from build123d import *

# Parameters (mm, degrees)
PROFILE_SKETCH_W               = 20
PROFILE_SKETCH_H               = 22
PROFILE_EXTRUDE_DEPTH          = 25
GUSSET_1_EXTRUDE_DEPTH         = 3
GUSSET_START                   = 22
GUSSET_2_EXTRUDE_DEPTH         = 3
SOLENOID_MOUNTING_HOLES_D      = 3.4
SOLENOID_MOUNTING_HOLES_DEPTH  = 3
NO_6_MOUNTING_HOLES_AT_2_COUNT = 2
NO_6_MOUNTING_HOLES_AT_2_PITCH = 10
FILLET3_R                      = 3
FILLET4_R                      = 2
FILLET5_R                      = 3
FILLET6_R                      = 1.5


with BuildPart() as part:
    # Profile Sketch → Profile  Extrude (new body)
    with BuildSketch(Plane.XY):
        Polygon((0, 0), (0, 25), (-26, 25), (-26, -4), (14, -4), (14, 0), align=None)
        with Locations((-13, 11)):
            Rectangle(PROFILE_SKETCH_W, PROFILE_SKETCH_H, mode=Mode.SUBTRACT)
    extrude(amount=PROFILE_EXTRUDE_DEPTH)

    # Gusset Sketch → Gusset 1 Extrude (add)
    with BuildSketch(Plane.XY):
        Polygon((0, 0), (14, 0), (0, 9), align=None)
    extrude(amount=GUSSET_1_EXTRUDE_DEPTH)

    # Gusset Sketch<2> → Gusset 2 Extrude (add)
    with BuildSketch(Plane.XY.offset(GUSSET_START)):
        Polygon((0, 0), (14, 0), (0, 9), align=None)
    extrude(amount=GUSSET_2_EXTRUDE_DEPTH)

    # Solenoid Mounting Holes
    with Locations(Plane(origin=(-25, 25, 0), x_dir=(0, 0, -1), z_dir=(0, 1, 0))):
        with Locations((-5, -17), (-20, -17), (-20, -7), (-5, -7)):
            Hole(SOLENOID_MOUNTING_HOLES_D / 2, depth=SOLENOID_MOUNTING_HOLES_DEPTH)

    # No. 6 Mounting Holes Profile Sketch → No. 6 Mounting Holes (revolve, cut)
    with BuildSketch(Plane(origin=(7, 0, 17.5), x_dir=(0, 0, 1), z_dir=(1, 0, 0))):
        Polygon((0, 0), (0, 4), (1.89865, 4), (1.89865, 1.891953401), (3.5433, 0), align=None)
    no_6_mounting_holes = revolve(axis=Axis((7, 6.35, 17.5), (0, -1, 0)), mode=Mode.SUBTRACT)

    # No. 6 Mounting Holes at 2: No. 6 Mounting Holes ×2
    with Locations(*[(0, 0, -i * NO_6_MOUNTING_HOLES_AT_2_PITCH) for i in range(1, NO_6_MOUNTING_HOLES_AT_2_COUNT)]):
        add(no_6_mounting_holes, mode=Mode.SUBTRACT)

    # Fillet3
    fillet3_edges = [part.edges().sort_by_distance(p)[0] for p in [
        (0, 9, 1.5),
        (0, 9, 23.5),
    ]]
    fillet(fillet3_edges, radius=FILLET3_R)

    # Fillet4
    fillet4_edges = [part.edges().sort_by_distance(p)[0] for p in [
        (14, 0, 12.5),
        (0, 0, 12.5),
    ]]
    fillet(fillet4_edges, radius=FILLET4_R)

    # Fillet5
    fillet5_edges = [part.edges().sort_by_distance(p)[0] for p in [
        (14, 0, 23.5),
        (14, 0, 1.5),
    ]]
    fillet(fillet5_edges, radius=FILLET5_R)

    # Fillet6
    fillet6_edges = [part.edges().sort_by_distance(p)[0] for p in [
        (-26, 25, 12.5),
        (0, 25, 12.5),
    ]]
    fillet(fillet6_edges, radius=FILLET6_R)


solid = part.part
The model under review builds one solid part; all positions refer to its coordinate system, in mm. A direction names the side the tool comes from. Give positions to 0.01 mm unless a question says otherwise; leave off trailing zeros. Write each loop counter-clockwise with the first axis right and the second up, starting at its lowest first coordinate (ties: lowest second). Pieces come first, ordered by that corner, then holes. Notation, with made-up numbers: M 46.25,7 L 52.25,7 A27 cw 52.25,31 Z; hole C 31,61 d8. An arc over 180 degrees is marked long. One line per question, with ' | ' between items. Start each with the question number.
Item 1: We need section D-D on y = 6.75. Write out the cut boundary in (x, z).
Item 2: We need section C-C on z = 1.5. Write out the cut boundary in (x, y), plus the area to 3 significant figures.
Item 3: We need section B-B on x = 7. Write out the cut boundary in (y, z), plus the area to 3 significant figures.
Item 4: For faces 1 (the flat face through (5, 3, 3)), 2 (the cylindrical face through (-19.433, 23.479, 5.914)), 3 (the cylindrical face through (13.643, -0.219, 23.521)), 4 (the flat face through (-13, 0, 12)), list the 3-axis set-ups (+Z, -Z, +X, -X, +Y, -Y) from which the entire face can be reached by the end or side of a thin tool; tool diameter is ignored.
Item 5: For pin 1 (4 mm diameter, centred on x = 5.5, y = 6, fed in from +Z); pin 2 (3 mm diameter, centred on x = -8, z = 20, fed in from +Y); pin 3 (6.5 mm diameter, centred on y = 7.5, z = 16, fed in from +X), all flat-tipped, find the tip position at first contact; note any pin that passes through.
Item 6: Draft analysis for pull direction Z (two halves, no side actions). For faces 5 (the cylindrical face through (-0.43, 24.55, 12.68)), 6 (the flat face through (-2, 7, 25)), 7 (the flat face through (5, 3, 22)), state which applies: released by +Z, released by -Z, zero draft, split by the parting line, or undercut.
Item 7: We need section A-A on z = 17.5. Write out the cut boundary in (x, y).
Item 8: Wall thickness on line 1 (Z direction, x = -8, y = 24.35); line 2 (Z direction, x = 7, y = -3.4); line 3 (Y direction, x = -7, z = 14): over which ranges is each line inside the solid? List them lowest first. Write a range as from..to.
Results found:
1) outline: M -26,0 L -23,0 L -23,25 L -26,25 Z; M -3,0 L 3.5,0 L 3.5,3 L 0,3 L 0,22 L 3.5,22 L 3.5,25 L -3,25 Z
2) outline: M -26,-4 L 14,-4 L 14,-1.64 A3 ccw 12.62,0.89 L 1.38,8.11 A3 cw 0,10.64 L 0,23.5 A1.5 ccw -1.5,25 L -24.5,25 A1.5 ccw -26,23.5 Z; hole M -23,0 L -3,0 L -3,22 L -23,22 Z | area: 432 mm2
3) outline: M -4,0 L 4.5,0 L 4.5,3 L 0,3 L 0,3.96 L -1.89,5.6 L -4,5.6 Z; M -4,9.4 L -1.89,9.4 L 0,11.04 L 0,13.96 L -1.89,15.6 L -4,15.6 Z; M -4,19.4 L -1.89,19.4 L 0,21.04 L 0,22 L 4.5,22 L 4.5,25 L -4,25 Z | area: 90.4 mm2
4) face 1: +X, +Y | face 2: +Y | face 3: +Z, -Z, +X, +Y | face 4: +Z, -Z
5) pin 1: stops at z = 25 | pin 2: stops at y = 0 | pin 3: stops at x = 0
6) face 5: zero draft | face 6: released by +Z | face 7: undercut
7) outline: M -26,-4 L 5.1,-4 L 5.1,-1.89 L 3.46,0 L 2,0 A2 cw 0,2 L 0,23.5 A1.5 ccw -1.5,25 L -24.5,25 A1.5 ccw -26,23.5 Z; M 8.9,-4 L 14,-4 L 14,-2 A2 ccw 12,0 L 10.54,0 L 8.9,-1.89 Z; hole M -23,0 L -3,0 L -3,22 L -23,22 Z
8) line 1: z = 0..3.3, 6.7..18.3, 21.7..25 | line 2: z = 0..5.6, 9.4..15.6, 19.4..25 | line 3: y = -4..0, 22..25
